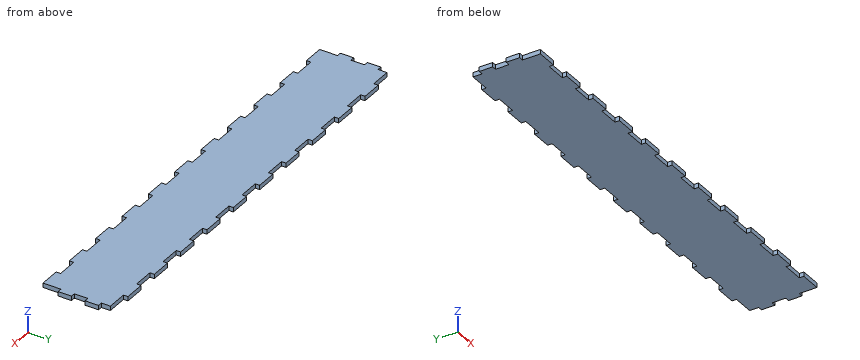
Autodesk Inventor part; units mm, degrees
ref_plane "YZ Plane" through (0, 0, 0) normal (1, 0, 0) x (0, 1, 0)
ref_plane "XZ Plane" through (0, 0, 0) normal (0, 1, 0) x (-1, 0, 0)
ref_plane "XY Plane" through (0, 0, 0) normal (0, 0, 1) x (1, 0, 0)
ref_plane "Work Plane1" through (139.4467, 111.518, -98.9659) normal (0, 0, -1) x (-1, 0, 0)
sketch "Sketch1" plane through (139.4467, 111.518, -98.9659) normal (0, 0, -1) x (-1, 0, 0)
  line L0 (0, -27.375) -> (14, -27.375)
  line L1 (14, -27.375) -> (14, -24.375)
  line L2 (14, -24.375) -> (28, -24.375)
  line L3 (28, -24.375) -> (28, -27.375)
  line L4 (56, -24.375) -> (56, -27.375)
  line L5 (42, -24.375) -> (56, -24.375)
  line L6 (42, -27.375) -> (42, -24.375)
  line L7 (28, -27.375) -> (42, -27.375)
  line L8 (84, -24.375) -> (84, -27.375)
  line L9 (70, -24.375) -> (84, -24.375)
  line L10 (70, -27.375) -> (70, -24.375)
  line L11 (56, -27.375) -> (70, -27.375)
  line L12 (112, -24.375) -> (112, -27.375)
  line L13 (98, -24.375) -> (112, -24.375)
  line L14 (98, -27.375) -> (98, -24.375)
  line L15 (84, -27.375) -> (98, -27.375)
  line L16 (140, -24.375) -> (140, -27.375)
  line L17 (126, -24.375) -> (140, -24.375)
  line L18 (126, -27.375) -> (126, -24.375)
  line L19 (112, -27.375) -> (126, -27.375)
  line L20 (168, -24.375) -> (168, -27.375)
  line L21 (154, -24.375) -> (168, -24.375)
  line L22 (154, -27.375) -> (154, -24.375)
  line L23 (140, -27.375) -> (154, -27.375)
  line L24 (196, -24.375) -> (196, -27.375)
  line L25 (182, -24.375) -> (196, -24.375)
  line L26 (182, -27.375) -> (182, -24.375)
  line L27 (168, -27.375) -> (182, -27.375)
  line L28 (224, -24.375) -> (224, -27.375)
  line L29 (210, -24.375) -> (224, -24.375)
  line L30 (210, -27.375) -> (210, -24.375)
  line L31 (196, -27.375) -> (210, -27.375)
  line L32 (252, -24.375) -> (252, -27.375)
  line L33 (238, -24.375) -> (252, -24.375)
  line L34 (238, -27.375) -> (238, -24.375)
  line L35 (224, -27.375) -> (238, -27.375)
  line L36 (280, -24.375) -> (280, -27.375)
  line L37 (266, -24.375) -> (280, -24.375)
  line L38 (266, -27.375) -> (266, -24.375)
  line L39 (252, -27.375) -> (266, -27.375)
  line L40 (280, -27.375) -> (294, -27.375)
  line L41 (0, 18.25) -> (14, 18.25)
  line L42 (14, 18.25) -> (14, 21.25)
  line L43 (14, 21.25) -> (28, 21.25)
  line L44 (28, 21.25) -> (28, 18.25)
  line L45 (56, 21.25) -> (56, 18.25)
  line L46 (42, 21.25) -> (56, 21.25)
  line L47 (42, 18.25) -> (42, 21.25)
  line L48 (28, 18.25) -> (42, 18.25)
  line L49 (84, 21.25) -> (84, 18.25)
  line L50 (70, 21.25) -> (84, 21.25)
  line L51 (70, 18.25) -> (70, 21.25)
  line L52 (56, 18.25) -> (70, 18.25)
  line L53 (112, 21.25) -> (112, 18.25)
  line L54 (98, 21.25) -> (112, 21.25)
  line L55 (98, 18.25) -> (98, 21.25)
  line L56 (84, 18.25) -> (98, 18.25)
  line L57 (140, 21.25) -> (140, 18.25)
  line L58 (126, 21.25) -> (140, 21.25)
  line L59 (126, 18.25) -> (126, 21.25)
  line L60 (112, 18.25) -> (126, 18.25)
  line L61 (168, 21.25) -> (168, 18.25)
  line L62 (154, 21.25) -> (168, 21.25)
  line L63 (154, 18.25) -> (154, 21.25)
  line L64 (140, 18.25) -> (154, 18.25)
  line L65 (196, 21.25) -> (196, 18.25)
  line L66 (182, 21.25) -> (196, 21.25)
  line L67 (182, 18.25) -> (182, 21.25)
  line L68 (168, 18.25) -> (182, 18.25)
  line L69 (224, 21.25) -> (224, 18.25)
  line L70 (210, 21.25) -> (224, 21.25)
  line L71 (210, 18.25) -> (210, 21.25)
  line L72 (196, 18.25) -> (210, 18.25)
  line L73 (252, 21.25) -> (252, 18.25)
  line L74 (238, 21.25) -> (252, 21.25)
  line L75 (238, 18.25) -> (238, 21.25)
  line L76 (224, 18.25) -> (238, 18.25)
  line L77 (280, 21.25) -> (280, 18.25)
  line L78 (266, 21.25) -> (280, 21.25)
  line L79 (266, 18.25) -> (266, 21.25)
  line L80 (252, 18.25) -> (266, 18.25)
  line L81 (280, 18.25) -> (294, 18.25)
  line L82 (297, 12.125) -> (297, 3)
  line L83 (297, 3) -> (294, 3)
  line L84 (294, 3) -> (294, -6.125)
  line L85 (297, -6.125) -> (294, -6.125)
  line L86 (297, -6.125) -> (297, -15.25)
  line L87 (297, -15.25) -> (294, -15.25)
  line L88 (294, -15.25) -> (294, -24.375)
  line L89 (297, 12.125) -> (294, 12.125)
  line L90 (0, -15.25) -> (0, -24.375)
  line L91 (0, -15.25) -> (-3, -15.25)
  line L92 (-3, -6.125) -> (-3, -15.25)
  line L93 (0, -6.125) -> (-3, -6.125)
  line L94 (0, 3) -> (0, -6.125)
  line L95 (0, 3) -> (-3, 3)
  line L96 (-3, 12.125) -> (-3, 3)
  line L97 (0, 12.125) -> (-3, 12.125)
  line L98 (0, -27.375) -> (0, -24.375)
  line L99 (0, 12.125) -> (0, 18.25)
  line L100 (294, -27.375) -> (294, -24.375)
  line L101 (294, 12.125) -> (294, 18.25)
  line L102 (294, 21.25) -> (-3, 21.25)
  point P0 (139.4467, -111.518)
  point P1 (28, -27.375)
  point P2 (56, -27.375)
  point P3 (168, -27.375)
  point P4 (224, -27.375)
  point P5 (252, 18.25)
  point P6 (224, 18.25)
  point P7 (196, 18.25)
  point P8 (168, 18.25)
  point P9 (140, 18.25)
  point P10 (112, 18.25)
  point P11 (84, 18.25)
  point P12 (56, 18.25)
  point P13 (28, 18.25)
  dimension "d0" = 3
  dimension "d1" = 14
  dimension "d4" = 28
  dimension "d13" = 3
  dimension "d14" = 14
  dimension "d15" = 28
extrude "Extrusion1" add sketch "Sketch1" along normal blind 3 contours L98 L90 L91 L92 L93 L94 L95 L96 L97 L99 L41 L42 L43 L44 L48 L47 L46 L45 L52 L51 L50 L49 L56 L55 L54 L53 L60 L59 L58 L57 L64 L63 L62 L61 L68 L67 L66 L65 L72 L71 L70 L69 L76 L75 L74 L73 L80 L79 L78 L77 L81 L101 L89 L82 L83 L84 L85 L86 L87 L88 L100 L40 L36 L37 L38 L39 L32 L33 L34 L35 L28 L29 L30 L31 L24 L25 L26 L27 L20 L21 L22 L23 L16 L17 L18 L19 L12 L13 L14 L15 L8 L9 L10 L11 L4 L5 L6 L7 L3 L2 L1 L0
properties part number "BackWall"
Model file for the job. Use its own axes, mm. Coordinates: 2 decimals unless noted, no trailing zeros. Order: outer loops, then holes, each group sorted by start corner. A loop starts at its lowest first (then second) coordinate and runs counter-clockwise, first axis right, second up. Notation, with made-up numbers: M 50.25,-7.75 L 89.25,-7.75 A9 cw 89.25,8.25 Z; hole C 19.25,-21.75 d3. An arc over 180 degrees is marked long. Answer as CSV lines item,"result".
(1) Wall check: line 1 along X through (y, z) = (126.5, -100.05); line 2 along Y through (x, z) = (16, -99.1); line 3 along Y through (x, z) = (-17.5, -100). Give the ranges that are in metal, low to high.
Geometry says:
line 1,"x = -154.55 to 139.45"
line 2,"y = 84.14 to 129.77"
line 3,"y = 87.14 to 132.77"
(2) Band-saw the part on B-B, the plane x = -108. List the corners of the cut face in (y, z), then the cut area to 3 significant figures.
Geometry says:
outline,"M 87.14,-101.97 L 132.77,-101.97 L 132.77,-98.97 L 87.14,-98.97 Z"
area,"137 mm2"
(3) Flat gauge pins, fed straight in: pin 1 (1.5 mm diameter, centred on x = 33.5, z = -100.5, fed in from -Y); pin 2 (1.5 mm diameter, centred on x = 141, z = -100, fed in from -Y); pin 3 (0.9 mm diameter, centred on y = 86.5, z = -101, fed in from +X). Where does each tip first touch, or does it go through?
Geometry says:
pin 1,"stops at y = 87.14"
pin 2,"stops at y = 96.27"
pin 3,"stops at x = 139.45"
(4) Band-saw the part on A-A, the plane y = 126.5. List the corners of the cut face in (x, z), then the cut area to 3 significant figures.
Geometry says:
outline,"M -154.55,-101.97 L 139.45,-101.97 L 139.45,-98.97 L -154.55,-98.97 Z"
area,"882 mm2"
